Could you check a few things on this drawing? It's one solid part, dimensions in mm from its lowest x, y, z. A direction names the side the tool comes from. Give positions to 0.01 mm unless a question says otherwise; leave off trailing zeros. Loops run counter-clockwise (first coordinate to the right, second up) from the corner with the lowest first, then second, coordinate; pieces in that order, holes last.
1. Imagine slicing it at D-D (y = 9). List the corners of the cut face in (x, z) for me.
2. I need wall thicknesses on line 1 along Y through (x, z) = (21.5, 6); line 2 along X through (y, z) = (7.5, 12.5); line 3 along X through (y, z) = (8.5, 9.5). Which ranges of each line are inside material? Lowest first, please.
3. Imagine slicing it at B-B (z = 14.5). List the corners of the cut face in (x, y) for me.
4. For P1, Ø0.6, axis at y = 1.5, z = 16, coming from the -X side; P2, Ø3, axis at x = 17.5, z = 12.5, coming from the +Y side; P3, Ø1.5, axis at x = 7, y = 3, coming from the +Z side, each with a flat end and sliding along its axis, tell me the tip position at first contact or that it passes through.
5. For the marked faces 5, 6 and 7, which set-ups out of +Z, -Z, +X, -X, +Y, -Y let a thin tool reach every point of the face, with its end or its side?
6. Thinking about a two-plate mould opening in Y: for the marked faces 1, 2, 3 and 4, which applies, +Y half, -Y half, draft (parallel to the pull), parting line (faces both ways), or undercut?
7. Imagine slicing it at C-C (z = 5). List the corners of the cut face in (x, y) for me, plus the area to 3 significant figures.
8. Imagine slicing it at A-A (x = 24). List the corners of the cut face in (y, z) for me.
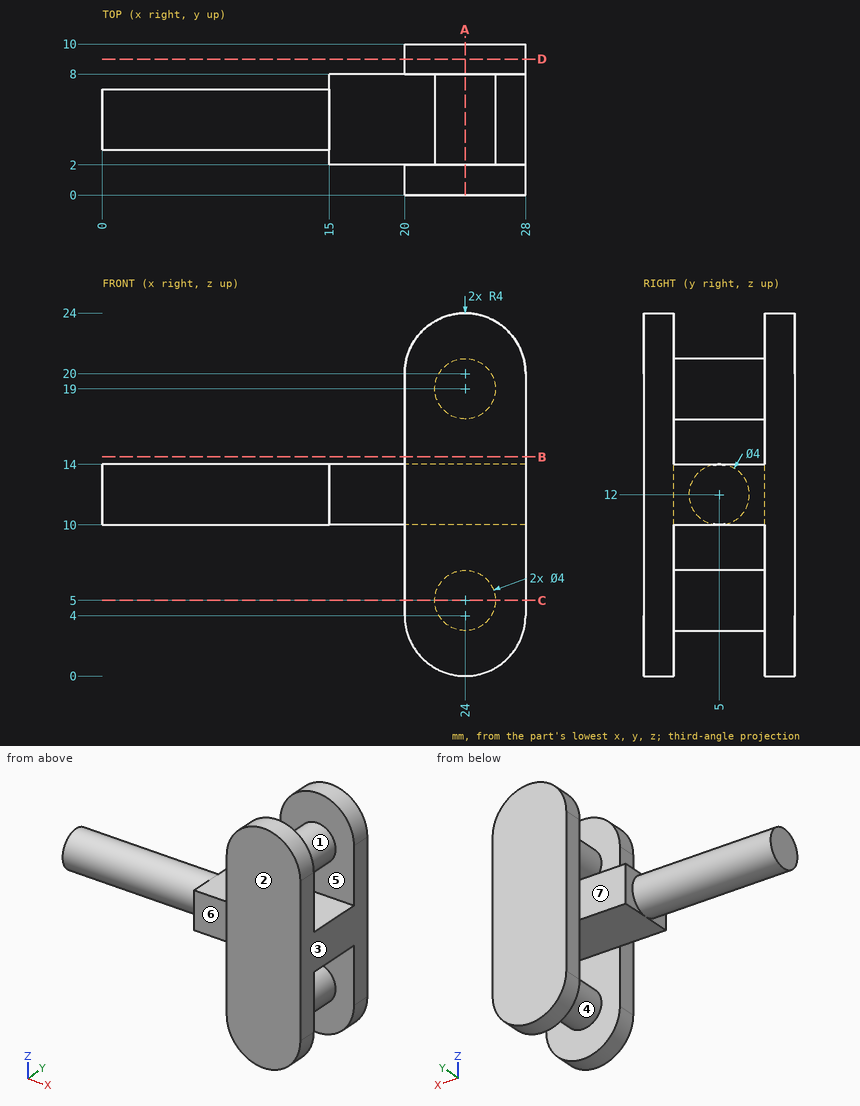
Derived:
1. outline: (20, 4) arc R4 ccw to (28, 4) - (28, 20) arc R4 ccw to (20, 20) - close
2. line 1: y = 0 to 2, 8 to 10
2. line 2: x = 15 to 28
2. line 3: x = 20 to 28
3. outline: (20, 0) - (28, 0) - (28, 2) - (20, 2) - close; (20, 8) - (28, 8) - (28, 10) - (20, 10) - close
4. P1: stops at x = 20
4. P2: stops at y = 8
4. P3: stops at z = 13.56
5. face 5: none
5. face 6: +Z, -Z, -X, -Y
5. face 7: +Z, -Z, -X, +Y
6. face 1: undercut
6. face 2: -Y half
6. face 3: draft
6. face 4: undercut
7. outline: (20, 0) - (28, 0) - (28, 2) - (26, 2) - (26, 8) - (28, 8) - (28, 10) - (20, 10) - (20, 8) - (22, 8) - (22, 2) - (20, 2) - close
7. area: 56.0 mm2
8. outline: (0, 0) - (2, 0) - (2, 3) - (8, 3) - (8, 0) - (10, 0) - (10, 24) - (8, 24) - (8, 21) - (2, 21) - (2, 24) - (0, 24) - close; hole (2, 7) - (8, 7) - (8, 10) - (2, 10) - close; hole (2, 14) - (8, 14) - (8, 17) - (2, 17) - close
